```python
from build123d import *

# Parameters (mm, degrees)
SKETCH1_W           = 52
SKETCH1_H           = 24
SKETCH1_R           = 8.25
BOSS_EXTRUDE1_DEPTH = 12
SKETCH2_R           = 1
CUT_EXTRUDE1_DEPTH  = 32.048349393
SKETCH3_R           = 1.75
CUT_EXTRUDE2_DEPTH  = 1
CUT_EXTRUDE3_DEPTH  = 5
FILLET3_R           = 0.5
CHAMFER1_SIZE       = 2.5
SKETCH5_W           = 14
SKETCH5_H           = 8
CUT_EXTRUDE4_DEPTH  = 5
FILLET4_R           = 0.5


with BuildPart() as part:
    # Sketch1 → Boss-Extrude1 (new body)
    with BuildSketch(Plane(origin=(0, 0, 0), x_dir=(1, 0, 0), z_dir=(0, 1, 0))):
        Rectangle(SKETCH1_W, SKETCH1_H)
        with Locations(Location((12.75, 0, 0), (0, 0, 270))):
            Circle(SKETCH1_R, mode=Mode.SUBTRACT)
        with Locations(Location((-12.75, 0, 0), (0, 0, 270))):
            Circle(SKETCH1_R, mode=Mode.SUBTRACT)
    extrude(amount=BOSS_EXTRUDE1_DEPTH)

    # Sketch2 → Cut-Extrude1 (cut, through all)
    with BuildSketch(Plane(origin=(0, 12, 0), x_dir=(1, 0, 0), z_dir=(0, 1, 0))):
        with Locations(Location((-21.35, 8.85, 0), (0, 0, 270))):
            Circle(SKETCH2_R)
        with Locations(Location((21.35, 8.85, 0), (0, 0, 270))):
            Circle(SKETCH2_R)
        with Locations(Location((21.35, -8.85, 0), (0, 0, 270))):
            Circle(SKETCH2_R)
        with Locations(Location((-21.35, -8.85, 0), (0, 0, 270))):
            Circle(SKETCH2_R)
    extrude(amount=-CUT_EXTRUDE1_DEPTH, mode=Mode.SUBTRACT)

    # Sketch3 → Cut-Extrude2 (cut)
    with BuildSketch(Plane(origin=(0, 12, 0), x_dir=(1, 0, 0), z_dir=(0, 1, 0))):
        with Locations(Location((-21.35, 8.85, 0), (0, 0, 270))):
            Circle(SKETCH3_R)
        with Locations(Location((21.35, 8.85, 0), (0, 0, 270))):
            Circle(SKETCH3_R)
        with Locations(Location((21.35, -8.85, 0), (0, 0, 270))):
            Circle(SKETCH3_R)
        with Locations(Location((-21.35, -8.85, 0), (0, 0, 270))):
            Circle(SKETCH3_R)
    extrude(amount=-CUT_EXTRUDE2_DEPTH, mode=Mode.SUBTRACT)

    # Sketch4 → Cut-Extrude3 (cut)
    with BuildSketch(Plane.XZ):
        Polygon((-6, -5), (-6, -12), (6, -12), (6, -5), (0, -5), align=None)
    extrude(amount=-CUT_EXTRUDE3_DEPTH, mode=Mode.SUBTRACT)

    # Fillet3
    fillet3_edges = [part.edges().sort_by_distance(p)[0] for p in [
        (-6, 2.5, -5),
        (6, 5, -8.5),
        (6, 2.5, -5),
        (-6, 5, -8.5),
        (0, 5, -5),
    ]]
    fillet(fillet3_edges, radius=FILLET3_R)

    # Chamfer1
    chamfer1_edges = [part.edges().sort_by_distance(p)[0] for p in [
        (26, 6, 12),
        (-26, 6, 12),
        (-26, 6, -12),
        (26, 6, -12),
    ]]
    chamfer(chamfer1_edges, length=CHAMFER1_SIZE)

    # Sketch5 → Cut-Extrude4 (cut)
    with BuildSketch(Plane.XZ):
        with Locations((0, 12)):
            Rectangle(SKETCH5_W, SKETCH5_H)
    extrude(amount=-CUT_EXTRUDE4_DEPTH, mode=Mode.SUBTRACT)

    # Fillet4
    fillet4_edges = [part.edges().sort_by_distance(p)[0] for p in [
        (-7, 2.5, 8),
        (7, 5, 10),
        (0, 5, 8),
        (-7, 5, 10),
        (7, 2.5, 8),
    ]]
    fillet(fillet4_edges, radius=FILLET4_R)


solid = part.part
```
CAD build for the part. Positions are in the model's coordinates, mm. A direction names the side the tool comes from. Coordinates: 2 decimals unless noted, no trailing zeros. Order: outer loops, then holes, each group sorted by start corner. A loop starts at its lowest first (then second) coordinate and runs counter-clockwise, first axis right, second up.
(1) Saw through at B-B, the plane y = 5.75. Write the cut outline in (x, z), and give its area (3 significant figures).
Solution:
outline: (-26, -9.5) - (-23.5, -12) - (23.5, -12) - (26, -9.5) - (26, 9.5) - (23.5, 12) - (-23.5, 12) - (-26, 9.5) - close; hole circle Ø2 at (-21.35, -8.85); hole circle Ø2 at (-21.35, 8.85); hole circle Ø16.5 at (-12.75, 0); hole circle Ø16.5 at (12.75, 0); hole circle Ø2 at (21.35, -8.85); hole circle Ø2 at (21.35, 8.85)
area: 795 mm2
(2) Pin check, flat tips, straight feed: pin 1 Ø4 at (x, z) = (-1, 10.5) entering from -Y; pin 2 Ø2.5 at (x, z) = (-21.35, -8.85) entering from +Y; pin 3 Ø10 at (x, z) = (12.75, 0) entering from -Y; pin 4 Ø3.5 at (x, y) = (2, 2.5) entering from -Z. Stop position of each tip, or through.
Solution:
pin 1: stops at y = 5
pin 2: stops at y = 11
pin 3: passes through
pin 4: stops at z = -5
(3) Saw through at D-D, the plane z = 0. Write the cut outline in (x, y), and give its area (3 significant figures).
Solution:
outline: (-26, 0) - (-21, 0) - (-21, 12) - (-26, 12) - close; (-4.5, 0) - (4.5, 0) - (4.5, 12) - (-4.5, 12) - close; (21, 0) - (26, 0) - (26, 12) - (21, 12) - close
area: 228 mm2
(4) Saw through at A-A, the plane z = -8.85. Write the cut outline in (x, y).
Solution:
outline: (-26, 0) - (-22.35, 0) - (-22.35, 11) - (-23.1, 11) - (-23.1, 12) - (-26, 12) - close; (-20.35, 0) - (-6, 0) - (-6, 4.5) arc R0.5 cw to (-5.5, 5) - (5.5, 5) arc R0.5 cw to (6, 4.5) - (6, 0) - (20.35, 0) - (20.35, 11) - (19.6, 11) - (19.6, 12) - (-19.6, 12) - (-19.6, 11) - (-20.35, 11) - close; (22.35, 0) - (26, 0) - (26, 12) - (23.1, 12) - (23.1, 11) - (22.35, 11) - close
(5) Drill centre lines: L1, parallel to X at y = 3.75, z = 0.25; L2, parallel to X at y = 11.4, z = 8.85; L3, parallel to X at y = 4, z = -8.5. Where is each one in solid material? Low to high.
Solution:
L1: x = -26 to -21, -4.5 to 4.5, 21 to 26
L2: x = -26 to -23.1, -19.6 to 19.6, 23.1 to 26
L3: x = -26 to -22.29, -20.41 to -6, 6 to 20.41, 22.29 to 26
(6) Which spindle directions (+Z, -Z, +X, -X, +Y, -Y) get a long thin tool onto all of the face, cutting with end or side? Do faces 4 (the face through (-23.06, 11.51, -9.23)), 5 (the face through (24.8, 5.9, -10.7)), 6 (the face through (7, 2, 10)), 7 (the face through (6, 2, -9)). Say none if no direction does.
Solution:
face 4: +Y
face 5: -Z, +X, +Y, -Y
face 6: +Z, -Y
face 7: -Z, -Y
(7) Saw through at C-C, the plane x = -12.75. Write the cut outline in (y, z).
Solution:
outline: (0, -12) - (12, -12) - (12, -8.25) - (0, -8.25) - close; (0, 8.25) - (12, 8.25) - (12, 12) - (0, 12) - close
(8) Mould opens along Z. For faces 1 (the face through (-22.5, 11, -8.9)), 2 (the face through (0, 12, 0)), 3 (the face through (0, 6, 12)) say: released by +Z, released by -Z, zero draft, split by the parting line, or undercut.
Solution:
face 1: undercut
face 2: zero draft
face 3: released by +Z
